Autodesk Inventor part; units mm, degrees
ref_plane "YZ Plane" through (0, 0, 0) normal (1, 0, 0) x (0, 1, 0)
ref_plane "XZ Plane" through (0, 0, 0) normal (0, 1, 0) x (-1, 0, 0)
ref_plane "XY Plane" through (0, 0, 0) normal (0, 0, 1) x (1, 0, 0)
sketch "Эскиз1" plane through (0, 0, 0) normal (0, 1, 0) x (-1, 0, 0)
  line L0 (25, 30) -> (-25, 30)
  line L1 (-30, 25) -> (-30, -25)
  line L2 (-25, -30) -> (25, -30)
  line L3 (30, -25) -> (30, 25)
  line L4 (0, -43.4497) -> (0, 43.4497)
  line L5 (-43.4497, 0) -> (43.4497, 0)
  arc A0 (30, 25) -> (25, 30) centre (25, 25) ccw
  arc A1 (25, -30) -> (30, -25) centre (25, -25) ccw
  arc A2 (-30, -25) -> (-25, -30) centre (-25, -25) ccw
  arc A3 (-25, 30) -> (-30, 25) centre (-25, 25) ccw
  circle A4 centre (25, 25) radius 5
  circle A5 centre (25, -25) radius 5
  circle A6 centre (-25, 25) radius 5
  circle A7 centre (-25, -25) radius 5
  point P0 (0, 0)
  dimension "d0" = 5
  dimension "d1" = 25
  dimension "d2" = 25
extrude "Выдавливание1" add sketch "Эскиз1" along normal blind 5 contours A4 L3 L5 L4 L0 | L4 L5 L1 A6 L0 | L5 L3 A5 L2 L4 | L4 L2 A7 L1 L5
extrude "Выдавливание2" add sketch "Эскиз1" along normal blind 50 contours A0 A4 | A6 A3 | A1 A5 | A2 A7
hole "Отверстие1" at (25, 0, 25) at (-25, 0, 25) at (25, 0, -25) at (-25, 0, -25) direction (0, 1, 0) diameter 4.134 depth 15 tip angle 118
sketch "Эскиз2" plane through (-25, 50, 25) normal (0, 1, 0) x (1, 0, 0)
  line L0 (-17, 25) -> (67, 25)
  line L1 (25, 67) -> (25, -17)
  point P0 (25, 25)
  point P1 (0.0023, -0.0231)
  point P2 (50.0023, -0.0231)
  point P3 (0.0023, 49.9769)
  point P4 (50.0023, 49.9769)
  dimension "d30" = 50
  dimension "d33" = 50
hole "Отверстие3" at (-24.9977, 50, 25.0231) at (-24.9977, 50, -24.9769) at (25.0023, 50, -24.9769) at (25.0023, 50, 25.0231) direction (0, -1, 0) diameter 4.134 depth 15 tip angle 118
properties part number "стойка для лотка"
Model file for the job. Use its own axes, mm. A direction names the side the tool comes from. Round coordinates to 2 decimals unless told otherwise and drop trailing zeros. Write each loop counter-clockwise with the first axis right and the second up, starting at its lowest first coordinate (ties: lowest second). Pieces come first, ordered by that corner, then holes. Notation, with made-up numbers: (43.5, 34.25) - (47.5, 34.25) arc R18 cw to (47.5, 66.25) - close; hole circle Ø7 at (50.5, 47). An arc over 180 degrees is marked (long way). One line per item, written item: value.
(1) Two-plate mould, pull along X, no slides. Class faces 4 (the flat face through (0, 2, -30)), 5 (the cylindrical face through (24.38, 7.6, 23.03)), 6 (the flat face through (30, 2, 0)): pulls with the +X half, pulls with the -X half, needs draft (parallel to the pull), parting line crosses it, or undercut.
Values follow:
face 4: needs draft
face 5: undercut
face 6: pulls with the +X half
(2) Cut at A-A, the plane y = 11.5. Give the cut face in (x, z).
Values follow:
outline: circle Ø10 at (-25, -25); circle Ø10 at (-25, 25); circle Ø10 at (25, -25); circle Ø10 at (25, 25); hole circle Ø4.13 at (-25, -25); hole circle Ø4.13 at (-25, 25); hole circle Ø4.13 at (25, -25); hole circle Ø4.13 at (25, 25)
(3) Wall check: probe 1 along X at (y, z) = (10, -25); probe 2 along Z at (x, y) = (-25, 4). Give the ranges that are in metal, low to high.
Values follow:
probe 1: x = -30 to -27.07, -22.93 to -20, 20 to 22.93, 27.07 to 30
probe 2: z = -30 to -27.07, -22.93 to 22.93, 27.07 to 30
(4) Drop flat-ended pins along their axis: P1, Ø5, axis at x = 25, z = 25.02, coming from the -Y side; P2, Ø3.5, axis at x = -25, z = -24.98, coming from the -Y side; P3, Ø12, axis at x = 18, y = 24.5, coming from the +Z side; P4, Ø18, axis at x = 2, z = 9.5, coming from the +Y side. Give the stop position or say it passes through.
Values follow:
P1: stops at y = 0
P2: stops at y = 15.18
P3: stops at z = 29.9
P4: stops at y = 5
(5) Cut at B-B, the plane y = 30.5. Give the cut face in (x, z), plus the area to 3 significant figures.
Values follow:
outline: circle Ø10 at (-25, -25); circle Ø10 at (-25, 25); circle Ø10 at (25, -25); circle Ø10 at (25, 25)
area: 314 mm²
(6) Cut at D-D, the plane z = 14. Give the cut face in (x, y).
Values follow:
outline: (-30, 0) - (30, 0) - (30, 5) - (-30, 5) - close
(7) Cut at C-C, the plane x = -13. Give the cut face in (y, z), plus the area to 3 significant figures.
Values follow:
outline: (0, -30) - (5, -30) - (5, 30) - (0, 30) - close
area: 300 mm²
(8) 3-axis set-ups, long thin cutter, end or side, ignore diameter. For faces 1 (the cylindrical face through (-25.62, 7.6, -26.97)), 2 (the flat face through (0, 0, 0)), 3 (the cylindrical face through (-27.307, 24.65, 29.436)): which of +Z, -Z, +X, -X, +Y, -Y reach the whole face in a straight line?
Values follow:
face 1: -Y
face 2: +Z, -Z, +X, -X, -Y
face 3: +Y
